Autodesk Inventor part; units mm, degrees
ref_plane "YZ Plane" through (0, 0, 0) normal (1, 0, 0) x (0, 1, 0)
ref_plane "XZ Plane" through (0, 0, 0) normal (0, 1, 0) x (-1, 0, 0)
ref_plane "XY Plane" through (0, 0, 0) normal (0, 0, 1) x (1, 0, 0)
sketch "Boceto1" plane through (0, 0, 0) normal (0, 0, 1) x (1, 0, 0)
  line L0 (-32.25, -14.25) -> (-32.25, 14.25)
  line L1 (-32.25, 14.25) -> (32.25, 14.25)
  line L2 (32.25, 14.25) -> (32.25, -14.25)
  line L3 (32.25, -14.25) -> (-32.25, -14.25)
  line L4 (34.25, 16.25) -> (-34.25, 16.25)
  line L5 (-34.25, 16.25) -> (-34.25, -16.25)
  line L6 (-34.25, -16.25) -> (34.25, -16.25)
  line L7 (34.25, -16.25) -> (34.25, 16.25)
  line L8 (32.25, -14.25) -> (32.25, -16.25)
  line L9 (32.25, 14.25) -> (32.25, 16.25)
  point P0 (0, 0)
  dimension "d0" = 2
extrude "Extrusión1" add sketch "Boceto1" along normal blind 2 and the other way blind 5 contours L3 L8 L6 L5 L4 L9 L1 L0 | L0 L1 L2 L3
shell "Vaciado1" thickness 2 removed faces 2 at (32.25, 5.4167, -0.3333) at (-12.0833, 5.4167, -5)
sketch "Boceto2" plane through (0, 0, -5) normal (0, 0, -1) x (-1, 0, 0)
  line L0 (-32.25, 14.25) -> (32.25, 14.25)
  line L1 (32.25, 14.25) -> (32.25, -14.25)
  line L2 (32.25, -14.25) -> (-32.25, -14.25)
  line L3 (-32.25, -14.25) -> (-32.25, -16.25)
  line L4 (-32.25, -16.25) -> (34.25, -16.25)
  line L5 (34.25, -16.25) -> (34.25, 16.25)
  line L6 (34.25, 16.25) -> (-32.25, 16.25)
  line L7 (-32.25, 16.25) -> (-32.25, 14.25)
  line L8 (-32.25, 16.25) -> (-24.25, 16.25)
  line L9 (-24.25, 16.25) -> (-24.25, 22.25)
  line L10 (-24.25, 22.25) -> (-32.25, 22.25)
  line L11 (-32.25, 22.25) -> (-32.25, 16.25)
  line L12 (-24.25, 22.25) -> (-32.25, 14.25)
  circle A0 centre (-28.25, 18.25) radius 2.1
  point P0 (0, 0)
  point P1 (-30.25, 16.25)
  point P2 (-29.7349, 16.7651)
  point P3 (-27.6097, 16.25)
  point P4 (-28.8903, 16.25)
  dimension "d6" = 8
  dimension "d7" = 6
  dimension "d8" = 4.2
extrude "Extrusión2" add sketch "Boceto2" against normal up to surface (7 mm away) contours L11 L10 L12 A0 L6 | L12 A0 L6 | L9 L6 A0 L12 picked at (-29.8223, 16.5215)
mirror "Simetría1" about plane through (0, 0, 0) normal (0, 1, 0) of "Extrusión2"
ref_plane "Plano de trabajo1" through (-1, -14.25, 0) normal (1, 0, 0) x (0, 0, -1)
mirror "Simetría2" about plane through (-1, -14.25, 0) normal (1, 0, 0) of "Extrusión2", "Simetría1"
fillet "Empalme1" radius 4 12 edges at (-26.25, 22.25, -1.5) (-34.25, 22.25, -1.5) (-34.25, -22.25, -1.5) (-26.25, -22.25, -1.5) (24.25, 22.25, -1.5) (32.25, 22.25, -1.5) (32.25, -22.25, -1.5) (24.25, -22.25, -1.5) (-26.25, 16.25, -1.5) (24.25, 16.25, -1.5) (24.25, -16.25, -1.5) (-26.25, -16.25, -1.5)
sketch "Boceto3" plane through (32.25, -14.25, 0) normal (0, 0, -1) x (-1, 0, 0)
  line L0 (64.5, 0) -> (64.5, 28.5)
  line L1 (64.5, 28.5) -> (0, 28.5)
  line L2 (0, 28.5) -> (0, 0)
  line L3 (0, 0) -> (64.5, 0)
  line L4 (64.5, 0) -> (0, 0)
  line L5 (0, 28.5) -> (57.5, 28.5)
  line L6 (57.5, 28.5) -> (57.5, 0)
  line L7 (57.5, 0) -> (0, 0)
  line L8 (0, 0) -> (0, 28.5)
  line L9 (54.5, 3) -> (54.5, 25.5)
  line L10 (57.5, 25.5) -> (0, 25.5)
  line L11 (3, 28.5) -> (3, 0)
  line L12 (0, 3) -> (57.5, 3)
  line L13 (2.55, 28.5) -> (2.55, 0)
  point P0 (32.25, 14.25)
  point P1 (57.5, 0)
  point P2 (2.55, 3)
  point P3 (2.55, 0)
  point P4 (2.55, 28.5)
  point P5 (2.55, 25.5)
  dimension "d12" = 57.5
  dimension "d13" = 3
  dimension "d16" = 0.45
extrude "Extrusión3" cut sketch "Boceto3" against normal blind 10 contours L3 L11 L12 L6 | L6 L10 L11 L1 | L3 L13 L12 L11 | L11 L10 L13 L1 | L3 L2 L12 L13 | L13 L10 L2 L1
properties part number "Soporte_ESP32S3"
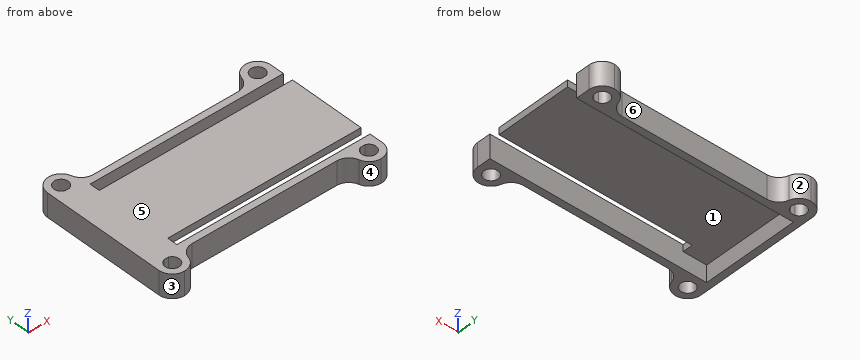
Build history of the part. All positions in model axes, mm. Face numbers are marked on the shaded views. A direction names the side the tool comes from. Round coordinates to 2 decimals unless told otherwise and drop trailing zeros. Write each loop counter-clockwise with the first axis right and the second up, starting at its lowest first coordinate (ties: lowest second). Pieces come first, ordered by that corner, then holes. Notation, with made-up numbers: M -27.5,-19.5 L -5.5,-19.5 A34 cw -5.5,17.5 Z; hole C 87.25,41 d9. An arc over 180 degrees is marked long. Answer as a JSON object with one key per item and string values. Group by question number.
(1) Drill centre lines: L1, parallel to Y at x = 28.25, z = -2.5; L2, parallel to Y at x = 4, z = 1.75; L3, parallel to Y at x = -15.5, z = -2.5. Where is each one in solid material? Low to high.
(2) Mould opens along X. For the marked faces 1, 2 and 3 say: pulls with the +X half, pulls with the -X half, needs draft (parallel to the pull), parting line crosses it, or undercut.
(3) Cut at A-A (x = 3). Give the cut face in (y, z), and give its area (3 significant figures).
(4) Flat gauge pins, fed straight in: pin 1 (14 mm diameter, centred on x = 15, y = 1.5, fed in from -Z); pin 2 (1 mm diameter, centred on x = -2, z = 0.5, fed in from +Y); pin 3 (0.6 mm diameter, centred on y = -12, z = 1, fed in from +X). Where does each tip first touch, or does it go through?
(5) Cut at C-C (z = -2.25). Give the number of separate pieces and of enclosed holes in the cut face, and give its area (3 significant figures).
(6) Cut at D-D (y = -13). Give the cut face in (x, z), and give its area (3 significant figures).
(7) Cut at B-B (y = 3). Give the cut face in (x, z), and give its area (3 significant figures).
(8) Which spindle directions (+Z, -Z, +X, -X, +Y, -Y) get a long thin tool onto all of the face, cutting with end or side? Do the marked faces 4, 5 and 6. Say none if no direction does.
Responses:
{
 "1": {"L1": "y = -22.25 to -20.35, -16.25 to -14.25, 14.25 to 16.25, 20.35 to 22.25", "L2": "y = -16.25 to -14.25, -11.25 to 11.25, 14.25 to 16.25", "L3": "y = -16.25 to -14.25, 14.25 to 16.25"},
 "2": {"face 1": "needs draft", "face 2": "undercut", "face 3": "pulls with the -X half"},
 "3": {"outline": "M -16.25,-5 L -14.25,-5 L -14.25,2 L -16.25,2 Z; M -11.25,0 L 11.25,0 L 11.25,2 L -11.25,2 Z; M 14.25,-5 L 16.25,-5 L 16.25,2 L 14.25,2 Z", "area": "73.0 mm2"},
 "4": {"pin 1": "stops at z = 0", "pin 2": "stops at y = 16.25", "pin 3": "stops at x = -25.25"},
 "5": {"separate pieces": "1", "enclosed holes": "4", "area": "443 mm2"},
 "6": {"outline": "M -34.25,-5 L -32.25,-5 L -32.25,0 L -25.25,0 L -25.25,2 L -34.25,2 Z", "area": "28.0 mm2"},
 "7": {"outline": "M -34.25,-5 L -32.25,-5 L -32.25,0 L 32.25,0 L 32.25,2 L -34.25,2 Z", "area": "143 mm2"},
 "8": {"face 4": "+Z, -Z, -Y", "face 5": "+Z, +X, -X, +Y, -Y", "face 6": "+Z, -Z, +Y"}
}
